```python
from build123d import *

# Parameters (mm, degrees)
SKETCH2_R               = 1.5
SKETCH2_R_2             = 1
BOSS_EXTRUDE2_DEPTH     = 5
SKETCH2_3_R             = 1.75
SKETCH2_3_R_2           = 1.5
BOSS_EXTRUDE3_DEPTH     = 0.333333333
SKETCH3_R               = 2
SKETCH3_R_2             = 1.5
BOSS_EXTRUDE4_DEPTH     = 0.333333333
SKETCH3_3_R             = 1.5
SKETCH3_3_R_2           = 1
BOSS_EXTRUDE5_DEPTH     = 1
SKETCH5_R               = 0.25
SKETCH5_W               = 0.5
SKETCH5_H               = 2.25
CUT_EXTRUDE1_DEPTH      = 2
CUT_EXTRUDE1_DEPTH_BACK = 2


with BuildPart() as part:
    # Sketch2 → Boss-Extrude2 (new body)
    with BuildSketch(Plane(origin=(0, 0, 0), x_dir=(1, 0, 0), z_dir=(0, 1, 0))):
        Circle(SKETCH2_R)
        Circle(SKETCH2_R_2, mode=Mode.SUBTRACT)
    extrude(amount=BOSS_EXTRUDE2_DEPTH)

    # Sketch2_3 → Boss-Extrude3 (add)
    with BuildSketch(Plane(origin=(0, 0, 0), x_dir=(1, 0, 0), z_dir=(0, 1, 0))):
        Circle(SKETCH2_3_R)
        Circle(SKETCH2_3_R_2, mode=Mode.SUBTRACT)
    extrude(amount=BOSS_EXTRUDE3_DEPTH)

    # Sketch3 → Boss-Extrude4 (add)
    with BuildSketch(Plane(origin=(0, 5, 0), x_dir=(-1, 0, 0), z_dir=(0, 1, 0))):
        Circle(SKETCH3_R)
        Circle(SKETCH3_R_2, mode=Mode.SUBTRACT)
    extrude(amount=-BOSS_EXTRUDE4_DEPTH)

    # Sketch3_3 → Boss-Extrude5 (add)
    with BuildSketch(Plane(origin=(0, 5, 0), x_dir=(-1, 0, 0), z_dir=(0, 1, 0))):
        Circle(SKETCH3_3_R)
        Circle(SKETCH3_3_R_2, mode=Mode.SUBTRACT)
    extrude(amount=BOSS_EXTRUDE5_DEPTH)

    # Sketch5 → Cut-Extrude1 (cut, two sides)
    with BuildSketch(Plane.XY) as cut_extrude1_sk:
        with Locations((0, 2.25)):
            Circle(SKETCH5_R)
        with Locations((0, 1.125)):
            Rectangle(SKETCH5_W, SKETCH5_H)
    extrude(amount=CUT_EXTRUDE1_DEPTH, mode=Mode.SUBTRACT)
    extrude(cut_extrude1_sk.sketch, amount=-CUT_EXTRUDE1_DEPTH_BACK, mode=Mode.SUBTRACT)


solid = part.part
```
The listing builds one solid part. Answer for the finished solid, in the listing's coordinates (mm). A direction names the side the tool comes from. Give positions to 0.01 mm unless a question says otherwise; leave off trailing zeros. Loops run counter-clockwise (first coordinate to the right, second up) from the corner with the lowest first, then second, coordinate; pieces in that order, holes last. Notation, with made-up numbers: (-1.5, 14) - (46.5, 14) arc R16 ccw to (46.5, 37) - close; hole circle Ø7 at (60.25, 32). An arc over 180 degrees is marked (long way). Return JSON: item names as keys, results as strings. Group by question number.
1. Which of the six approach directions +Z, -Z, +X, -X, +Y, -Y give full straight-line access (tool end or side, diameter ignored) to faces 1 (the cylindrical face through (1.5, 5.49, 0.07)), 2 (the cylindrical face through (-1.75, 0.16, -0.03)), 3 (the cylindrical face through (0.69, 2.47, 1.33))?
2. Find section C-C (y = 1.25). Write down the section's boundary in (x, z), then the cut area to 3 significant figures.
3. Given pin 1 Ø0.8 at (y, z) = (1.5, 1.5) entering from -X; pin 2 Ø2 at (x, y) = (1.5, 4.5) entering from -Z; pin 3 Ø1.5 at (x, y) = (-0.5, 3.5) entering from +Z, each flat-ended and moving along its own axis, determine where each tip first touches the part or whether it passes through.
4. Find section A-A (x = 0). Write down the section's boundary in (y, z), then the cut area to 3 significant figures.
5. Find section B-B (z = -0.15). Write down the section's boundary in (x, y), then the cut area to 3 significant figures.
6. Find section D-D (y = 4). Write down the section's boundary in (x, z), then the cut area to 3 significant figures.
7. Straight lines are drawn through the part: line 1 (Y direction, x = 1.1, z = 1.3); line 2 (Z direction, x = 0, y = 5.85). For each, find the intervals that lie inside material, in ascending order. Write a range as [from, to].
Verdict:
{
 "1": {"face 1": "+Y", "face 2": "-X, -Y", "face 3": "none"},
 "2": {"outline": "(-0.25, -1.48) - (-0.25, -0.97) arc R1 cw to (-0.25, 0.97) - (-0.25, 1.48) arc R1.5 ccw to start; (0.25, -1.48) arc R1.5 ccw to (0.25, 1.48) - (0.25, 0.97) arc R1 cw to (0.25, -0.97) - close", "area": "3.42 mm^2"},
 "3": {"pin 1": "stops at x = -1.02", "pin 2": "stops at z = -1.93", "pin 3": "stops at z = 1.5"},
 "4": {"outline": "(2.5, -1.5) - (4.67, -1.5) - (4.67, -2) - (5, -2) - (5, -1.5) - (6, -1.5) - (6, -1) - (2.5, -1) - close; (2.5, 1) - (6, 1) - (6, 1.5) - (5, 1.5) - (5, 2) - (4.67, 2) - (4.67, 1.5) - (2.5, 1.5) - close", "area": "3.83 mm^2"},
 "5": {"outline": "(-1.99, 4.67) - (-1.49, 4.67) - (-1.49, 0.33) - (-1.74, 0.33) - (-1.74, 0) - (-0.99, 0) - (-0.99, 6) - (-1.49, 6) - (-1.49, 5) - (-1.99, 5) - close; (0.99, 0) - (1.74, 0) - (1.74, 0.33) - (1.49, 0.33) - (1.49, 4.67) - (1.99, 4.67) - (1.99, 5) - (1.49, 5) - (1.49, 6) - (0.99, 6) - close", "area": "6.55 mm^2"},
 "6": {"outline": "circle Ø3 at (0, 0); hole circle Ø2 at (0, 0)", "area": "3.93 mm^2"},
 "7": {"line 1": "y = [0, 0.33], [4.67, 5]", "line 2": "z = [-1.5, -1], [1, 1.5]"}
}
